Here's how the part is built. I have some questions about the finished solid (model axes, mm). A direction names the side the tool comes from. Give positions to 0.01 mm unless a question says otherwise; leave off trailing zeros. Write each loop counter-clockwise with the first axis right and the second up, starting at its lowest first coordinate (ties: lowest second). Pieces come first, ordered by that corner, then holes. Notation, with made-up numbers: (-20, 0.25) - (-9, 0.25) arc R21 cw to (-9, 23.25) - close; hole circle Ø7 at (65, 20.25). An arc over 180 degrees is marked (long way). One line per item, written item: value. Start each with the question number.
1) On a 3-axis mill with a long thin cutter (end or side, diameter ignored), from which of +Z, -Z, +X, -X, +Y, -Y can I reach the whole of each face in a straight line? I mean faces 1 (the flat face through (0, 0, -4)), 2 (the flat face through (4, 2, 0)). Say none if no direction works.
2) Imagine slicing it at D-D on z = 15. Write out the boundary of the cut face in (x, y).
3) I'm going to push flat-ended pins straight in: P1, Ø3, axis at x = 5, y = 4.5, coming from the -Z side; P2, Ø3.5, axis at x = 4.5, z = 1, coming from the -Y side; P3, Ø2, axis at x = 5, z = -13, coming from the -Y side. Where does each tip first touch, or does it pass through?
4) Imagine slicing it at A-A on z = 0. Write out the boundary of the cut face in (x, y).
5) Imagine slicing it at B-B on y = 0. Write out the boundary of the cut face in (x, z).
6) We'd pull the mould along Z, two halves only. Please class faces 3 (the cylindrical face through (3.55, -12.273, -0.358)), 4 (the cylindrical face through (3.65, -0.88, -19.98)), 5 (the flat face through (7.2, 0, -4)): +Z half, -Z half, draft (parallel to the pull), parting line (faces both ways), or undercut.
7) Please list where these lines run through material, in increasing order: L1, parallel to Y at x = 3.5, z = 0; L2, parallel to Y at x = 3.5, z = 15; L3, parallel to Y at x = 5, z = -14. Write a range as [from, to].
8) Imagine slicing it at C-C on x = 1. Write out the boundary of the cut face in (y, z).
from build123d import *

# Parameters (mm, degrees)
ESBO_O1_W               = 7.2
ESBO_O1_H               = 20
CORTE_EXTRUS_O2_DEPTH   = 30.186298155
FURO_COM_FOLGA_DE_M51_D = 5.5


with BuildPart() as part:
    # Esboço1 → Revolução1 (revolve)
    with BuildSketch(Plane.XY, mode=Mode.PRIVATE) as revolu_o1_sk:
        with Locations((3.6, 10)):
            Rectangle(ESBO_O1_W, ESBO_O1_H)
    revolve(revolu_o1_sk.sketch.rotate(Axis((-35, 0, 0), (1, 0, 0)), 90), axis=Axis((-35, 0, 0), (1, 0, 0)))

    # Esboço3 → Corte-extrusão2 (cut, through all)
    with BuildSketch(Plane(origin=(7.2, 0, 0), x_dir=(0, 0, -1), z_dir=(1, 0, 0))):
        with BuildLine():
            Line((-2.236067977, 2), (2.236067977, 2))
            ThreePointArc((2.236067977, 2), (0, -3), (-2.236067977, 2))
        make_face()
    extrude(amount=-CORTE_EXTRUS_O2_DEPTH, mode=Mode.SUBTRACT)

    # Furo com folga de M51 (through all)
    with Locations(Plane(origin=(7.2, 0, 0), x_dir=(0, 0, -1), z_dir=(1, 0, 0))):
        with Locations((0, 15), (15, 0), (0, -15), (-15, 0)):
            Hole(FURO_COM_FOLGA_DE_M51_D / 2)


solid = part.part
Numbers:
1. face 1: +Z, -Z, -X, +Y, -Y
1. face 2: +X, -X
2. outline: (0, -13.23) - (7.2, -13.23) - (7.2, -2.75) - (0, -2.75) - close; (0, 2.75) - (7.2, 2.75) - (7.2, 13.23) - (0, 13.23) - close
3. P1: z = -19.77
3. P2: y = -20
3. P3: y = -16
4. outline: (0, -20) - (7.2, -20) - (7.2, -17.75) - (0, -17.75) - close; (0, -12.25) - (7.2, -12.25) - (7.2, -3) - (0, -3) - close; (0, 2) - (7.2, 2) - (7.2, 12.25) - (0, 12.25) - close; (0, 17.75) - (7.2, 17.75) - (7.2, 20) - (0, 20) - close
5. outline: (0, -20) - (7.2, -20) - (7.2, -17.75) - (0, -17.75) - close; (0, -12.25) - (7.2, -12.25) - (7.2, -3) - (0, -3) - close; (0, 3) - (7.2, 3) - (7.2, 12.25) - (0, 12.25) - close; (0, 17.75) - (7.2, 17.75) - (7.2, 20) - (0, 20) - close
6. face 3: undercut
6. face 4: parting line
6. face 5: draft
7. L1: [-20, -17.75], [-12.25, -3], [2, 12.25], [17.75, 20]
7. L2: [-13.23, -2.75], [2.75, 13.23]
7. L3: [-14.28, -2.56], [2.56, 14.28]
8. outline: circle Ø40 at (0, 0); hole circle Ø5.5 at (-15, 0); hole circle Ø5.5 at (0, -15); hole circle Ø5.5 at (0, 15); hole (2, -2.24) - (2, 2.24) arc R3 ccw (long way) to start; hole circle Ø5.5 at (15, 0)
